Autodesk Inventor part; units mm, degrees
ref_plane "YZ Plane" through (0, 0, 0) normal (1, 0, 0) x (0, 1, 0)
ref_plane "XZ Plane" through (0, 0, 0) normal (0, 1, 0) x (-1, 0, 0)
ref_plane "XY Plane" through (0, 0, 0) normal (0, 0, 1) x (1, 0, 0)
sketch "Sketch1" plane through (0, 0, 0) normal (0, 0, 1) x (1, 0, 0)
  circle A0 centre (0, 0) radius 10.685 construction
  line L0 (-0.9, 10.647) -> (-0.9, -10.647) construction
  line L1 (-0.9, 10.647) -> (20.3941, 10.647) construction
  arc A1 (-0.9, 15.1232) -> (-0.9, -15.1232) centre (0, 0) ccw
  line L2 (-0.9, 10.647) -> (-0.9, 15.1232)
  line L3 (-0.9, -15.1232) -> (-0.9, -10.647)
  arc A2 (-0.9, 10.647) -> (-0.9, -10.647) centre (0, 0) ccw
  dimension "d0" = 21.37
  dimension "d1" = 90
  dimension "d2" = 0.9
  dimension "d3" = 15.15
extrude "Extrusion1" add sketch "Sketch1" along normal blind 27
sketch "Sketch2" plane through (0, 0, 27) normal (0, 0, 1) x (1, 0, 0)
  arc A0 (-0.9, 17.627) -> (-0.9, -17.627) centre (0, 0) ccw
  arc A1 (-0.9, 15.1232) -> (-0.9, -15.1232) centre (0, 0) ccw
  line L0 (-0.9, 10.647) -> (-0.9, 15.1232)
  line L1 (-0.9, 10.647) -> (-0.9, 17.627)
  line L2 (-0.9, -17.627) -> (-0.9, -10.647)
  arc A2 (-0.9, 10.647) -> (-0.9, -10.647) centre (0, 0) ccw
  arc A3 (-0.9, 10.647) -> (-0.9, -10.647) centre (0, 0) ccw
  point P0 (-0.9, 15.1232)
  dimension "d6" = 17.65
extrude "Extrusion2" add sketch "Sketch2" along normal blind 2.6
properties part number "Shim"
Can you work these out from the model? Positions are in its coordinate system, mm. Give positions to 0.01 mm unless a question says otherwise; leave off trailing zeros. Loops run counter-clockwise (first coordinate to the right, second up) from the corner with the lowest first, then second, coordinate; pieces in that order, holes last. Notation, with made-up numbers: (10.5, 57) -> (17.5, 57) arc R24 ccw to (17.5, 94) -> close; hole circle Ø5 at (78, 34). An arc over 180 degrees is marked (long way). Return JSON: item names as keys, results as strings.
Q1. I want a section at A-A, the plane y = 0. List the corners of the cut face in (x, z) for me.
Checks:
{"outline": "(-17.65, 27) -> (-15.15, 27) -> (-15.15, 0) -> (-10.68, 0) -> (-10.68, 29.6) -> (-17.65, 29.6) -> close"}
Q2. I need wall thicknesses on probe 1 along Z at (x, y) = (-14.25, -6); probe 2 along Y at (x, z) = (-1.75, 21); probe 3 along Y at (x, z) = (-2.5, 19). Which ranges of each line are inside material? Lowest first, please.
Checks:
{"probe 1": "z = 27 to 29.6", "probe 2": "y = -15.05 to -10.54, 10.54 to 15.05", "probe 3": "y = -14.94 to -10.39, 10.39 to 14.94"}
Q3. We'd pull the mould along Y, two halves only. Please class faces 1 (the face through (-16, 0, 27)), 2 (the face through (-15.147, -0.321, 13.311)), 3 (the face through (-10.683, -0.222, 14.593)): released by +Y, released by -Y, zero draft, split by the parting line, or undercut.
Checks:
{"face 1": "zero draft", "face 2": "split by the parting line", "face 3": "undercut"}
Q4. I want a section at B-B, the plane x = -14.5. List the corners of the cut face in (y, z) for me, then the cut area to 3 significant figures.
Checks:
{"outline": "(-10.06, 27) -> (-4.39, 27) -> (-4.39, 0) -> (4.39, 0) -> (4.39, 27) -> (10.06, 27) -> (10.06, 29.6) -> (-10.06, 29.6) -> close", "area": "289 mm2"}
Q5. For pin 1 Ø1.5 at (x, z) = (-12.5, 7) entering from +Y; pin 2 Ø1 at (y, z) = (3.5, 9.5) entering from -X; pin 3 Ø2 at (x, z) = (-13.5, 19) entering from -Y, each with a flat end and sliding along its axis, tell me the tip position at first contact or that it passes through.
Checks:
{"pin 1": "stops at y = 9.56", "pin 2": "stops at x = -14.85", "pin 3": "stops at y = -8.56"}
Q6. I want a section at D-D, the plane y = 12.5. List the corners of the cut face in (x, z) for me.
Checks:
{"outline": "(-12.46, 27) -> (-8.56, 27) -> (-8.56, 0) -> (-0.9, 0) -> (-0.9, 29.6) -> (-12.46, 29.6) -> close"}
